Geometry check sheet. Reference: drawing and pictorial views, mm from the part's lowest x, y, z. A direction names the side the tool comes from. Give positions to 0.01 mm unless a question says otherwise; leave off trailing zeros. Write each loop counter-clockwise with the first axis right and the second up, starting at its lowest first coordinate (ties: lowest second). Pieces come first, ordered by that corner, then holes. Notation, with made-up numbers: (67, -37) -> (126, -37) arc R15 ccw to (126, -22) -> close; hole circle Ø5 at (39.25, -4). An arc over 180 degrees is marked (long way). Use a Markdown table: item, result. Add a question column.
1. Cross-section at D-D (z = 69.27). Enter the section's corners in (x, y), then the cut area to 3 significant figures.
2. Set-up check for the marked faces 1, 2 and 3: record each of +Z, -Z, +X, -X, +Y, -Y from which the full face is reachable in a straight line by a thin tool's end or side.
3. Gauge pin test, flat ends, axial feed: P1, Ø12, axis at x = 12.5, z = 8.5, coming from the -Y side; P2, Ø7.5, axis at y = 39, z = 69.27, coming from the -X side; P3, Ø12, axis at y = 70, z = 20, coming from the +X side; P4, Ø6, axis at x = 45.5, z = 52, coming from the +Y side. Record the tip position at first contact, or that the pin passes through.
4. Cross-section at A-A (z = 39). Enter the section's corners in (x, y), then the cut area to 3 significant figures.
5. Scan lines: probe 1 along Y at (x, z) = (48.75, 39); probe 2 along Y at (x, z) = (54.75, 39); probe 3 along X at (y, z) = (26.5, 69.5). Record each from-to range of solid material in increasing order. Write a range as [from, to].
6. Cross-section at B-B (y = 68). Enter the section's corners in (x, z), then the cut area to 3 significant figures.
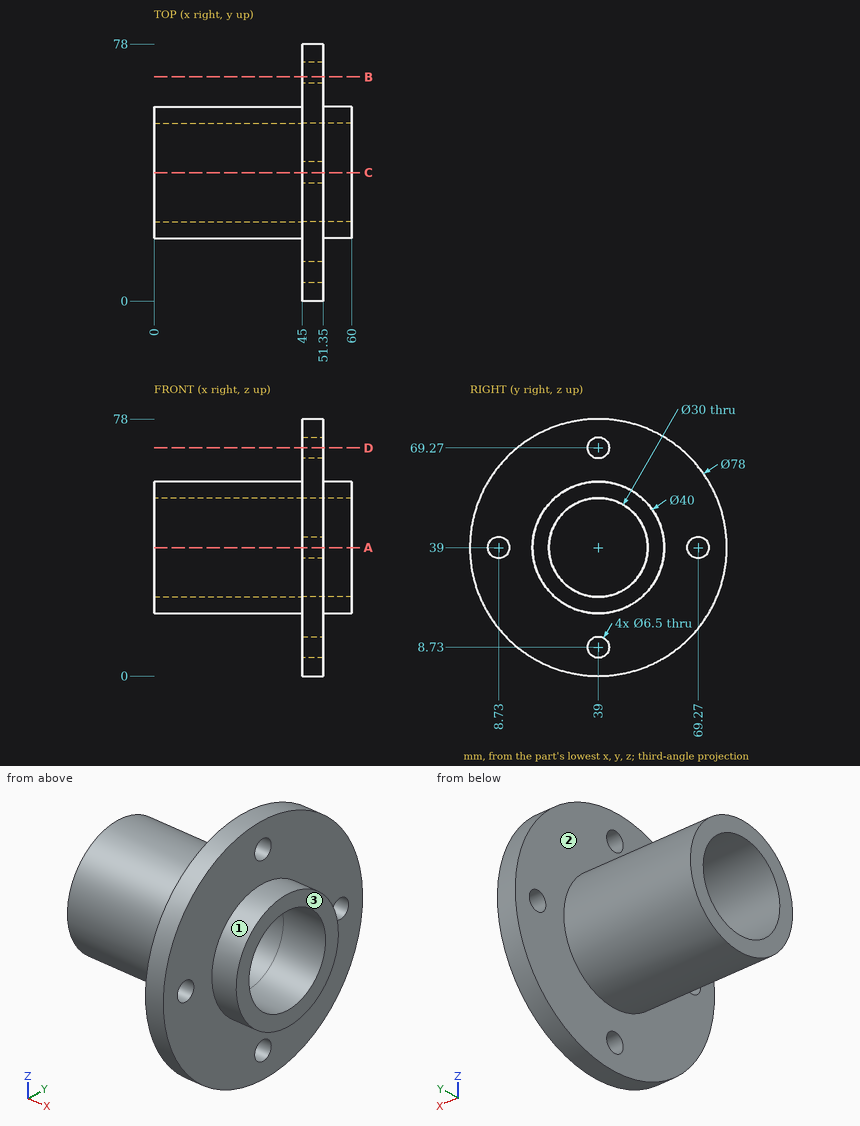
Worked answers:
| question | item | result |
|---|---|---|
| 1 | outline | (45, 14.41) -> (51.35, 14.41) -> (51.35, 35.75) -> (45, 35.75) -> close; (45, 42.25) -> (51.35, 42.25) -> (51.35, 63.59) -> (45, 63.59) -> close |
| 1 | area | 271 mm² |
| 2 | face 1 | +X |
| 2 | face 2 | -X |
| 2 | face 3 | +Z, -Z, +X, +Y, -Y |
| 3 | P1 | passes through |
| 3 | P2 | stops at x = 45 |
| 3 | P3 | stops at x = 51.35 |
| 3 | P4 | stops at y = 76.7 |
| 4 | outline | (0, 19) -> (45, 19) -> (45, 11.98) -> (51.35, 11.98) -> (51.35, 19) -> (60, 19) -> (60, 24) -> (0, 24) -> close; (0, 54) -> (60, 54) -> (60, 59) -> (51.35, 59) -> (51.35, 66.02) -> (45, 66.02) -> (45, 59) -> (0, 59) -> close; (45, 0) -> (51.35, 0) -> (51.35, 5.48) -> (45, 5.48) -> close; (45, 72.52) -> (51.35, 72.52) -> (51.35, 78) -> (45, 78) -> close |
| 4 | area | 759 mm² |
| 5 | probe 1 | y = [0, 5.48], [11.98, 24], [54, 66.02], [72.52, 78] |
| 5 | probe 2 | y = [19, 24], [54, 59] |
| 5 | probe 3 | x = [45, 51.35] |
| 6 | outline | (45, 12.92) -> (51.35, 12.92) -> (51.35, 36.01) -> (45, 36.01) -> close; (45, 41.99) -> (51.35, 41.99) -> (51.35, 65.08) -> (45, 65.08) -> close |
| 6 | area | 293 mm² |
